Could you check a few things on this model? Use its own coordinates, in mm. Face numbers are marked on the shaded views. A direction names the side the tool comes from. Coordinates: 2 decimals unless noted, no trailing zeros. Loops run counter-clockwise (first coordinate to the right, second up) from the corner with the lowest first, then second, coordinate; pieces in that order, holes last. Notation, with made-up numbers: M 31.25,-24 L 56.25,-24 A22 ccw 56.25,11 Z; hole C 62,21 d11. An arc over 180 degrees is marked long. Return JSON: item names as keys, results as strings. Group by question number.
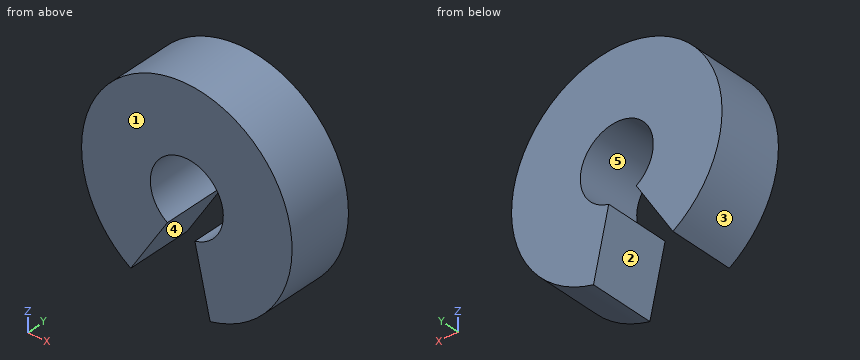
from build123d import *

# Parameters (mm, degrees)
SKETCH1_R           = 11.25
BOSS_EXTRUDE1_DEPTH = 7
SKETCH2_R           = 3.9
CUT_EXTRUDE1_DEPTH  = 7
CUT_EXTRUDE2_DEPTH  = 7


with BuildPart() as part:
    # Sketch1 → Boss-Extrude1 (new body)
    with BuildSketch(Plane(origin=(0, 0, 0), x_dir=(1, 0, 0), z_dir=(0, 1, 0))):
        with Locations(Location((0, 0, 0), (0, 0, 270))):
            Circle(SKETCH1_R)
    extrude(amount=BOSS_EXTRUDE1_DEPTH)

    # Sketch2 → Cut-Extrude1 (cut)
    with BuildSketch(Plane(origin=(0, 7, 0), x_dir=(1, 0, 0), z_dir=(0, 1, 0))):
        with Locations(Location((0, 0, 0), (0, 0, 270))):
            Circle(SKETCH2_R)
    extrude(amount=-CUT_EXTRUDE1_DEPTH, mode=Mode.SUBTRACT)

    # Sketch3 → Cut-Extrude2 (cut)
    with BuildSketch(Plane(origin=(0, 7, 0), x_dir=(1, 0, 0), z_dir=(0, 1, 0))):
        Polygon((-40.112737078, 63.658014265), (-5.997550022, 9.517977397), (0, 0), (2.48931807, 10.971134652), (16.649025164, 73.377001963), (-4.9506307, 199.525379622), (-61.712392941, 189.806391923), align=None)
    extrude(amount=-CUT_EXTRUDE2_DEPTH, mode=Mode.SUBTRACT)


solid = part.part
(1) We'd pull the mould along X, two halves only. Please class the marked faces 1, 2 and 3: +X half, -X half, draft (parallel to the pull), parting line (faces both ways), or undercut.
(2) Imagine slicing it at B-B, the plane y = 5.25. Write out the boundary of the cut face in (x, z).
(3) If I drill on L1, parallel to X at y = 3, z = 0; L2, parallel to Z at x = 0, y = 0.5; L3, parallel to X at y = 3.25, z = 2.25, over which ranges is the centre line in solid material (lowest first)? Write a range as [from, to].
(4) Imagine slicing it at D-D, the plane x = 0. Write out the boundary of the cut face in (y, z).
(5) For the marked faces 4 and 5, which set-ups out of +Z, -Z, +X, -X, +Y, -Y let a thin tool reach every point of the face, with its end or its side?
(6) Will these pins go through, and if not, where does the flat tip stop? P1, Ø3, axis at x = 5.5, y = 2.5, coming from the -Z side; P2, Ø2, axis at x = 1.5, y = 2, coming from the +Z side; P3, Ø4, axis at y = 2.5, z = 6, coming from the +X side.
(7) Imagine slicing it at A-A, the plane z = 0. Write out the boundary of the cut face in (x, y).
(8) Imagine slicing it at C-C, the plane z = 2.25. Write out the boundary of the cut face in (x, y).
Checks:
{
 "1": {"face 1": "draft", "face 2": "undercut", "face 3": "parting line"},
 "2": {"outline": "M -6,-9.52 L -2.08,-3.3 A3.9 cw long 0.86,-3.8 L 2.49,-10.97 A11.25 ccw long Z"},
 "3": {"L1": "[-11.25, -3.9], [3.9, 11.25]", "L2": "[3.9, 11.25]", "L3": "[-11.02, -3.19], [3.19, 11.02]"},
 "4": {"outline": "M 0,3.9 L 7,3.9 L 7,11.25 L 0,11.25 Z"},
 "5": {"face 4": "-Z, +Y, -Y", "face 5": "+Y, -Y"},
 "6": {"P1": "z = -10.51", "P2": "z = 11.24", "P3": "x = 10.51"},
 "7": {"outline": "M -11.25,0 L -3.9,0 L -3.9,7 L -11.25,7 Z; M 3.9,0 L 11.25,0 L 11.25,7 L 3.9,7 Z"},
 "8": {"outline": "M -11.02,0 L -3.19,0 L -3.19,7 L -11.02,7 Z; M 3.19,0 L 11.02,0 L 11.02,7 L 3.19,7 Z"}
}
